from build123d import *

# Parameters (mm, degrees)
F2_W           = 143.0530622602
F2_H           = 41.3108188659
F3_DEPTH       = 14.2
F4_DEPTH       = 45
F5_R           = 3.175
F6_DEPTH       = 25
F7_R           = 11.27
F7_R_2         = 5.0034619329
F8_DEPTH       = 20.6
F9_DEPTH       = 38.1921002041
F11_R          = 5.5610063416
F12_DEPTH      = 13
F13_R          = 3.175
F14_DEPTH      = 25.5131088414
F14_DEPTH_BACK = 25


with BuildPart() as f1:
    # F0 (on Front) → F1 (revolve)
    with BuildSketch(Plane.XZ):
        with BuildLine():
            ThreePointArc((-23.8617697281, 6.3559776459), (-20.6996107179, 0.4699326202), (-16.1176094264, -4.3931980396))
            Line((-16.1176094264, -4.3931980396), (-16.1176094264, 11.4784657965))
            Line((-16.1176094264, 11.4784657965), (0, 11.4784657965))
            Line((0, 11.4784657965), (0, 40.8949155528))
            ThreePointArc((0, 40.8949155528), (-20.9900112333, 29.8840868605), (-23.8617697281, 6.3559776459))
        make_face()
        with BuildLine():
            ThreePointArc((-16.1176094264, -4.3931980396), (-8.5539497274, -8.6525348005), (0, -10.12930213))
            Line((0, -10.12930213), (0, 11.4784657965))
            Line((0, 11.4784657965), (-16.1176094264, 11.4784657965))
            Line((-16.1176094264, 11.4784657965), (-16.1176094264, -4.3931980396))
        make_face()
        with BuildLine():
            Line((-16.1176094264, -14.11514998), (-16.1176094264, -39.7087657565))
            Line((-16.1176094264, -39.7087657565), (0, -39.7087657565))
            Line((0, -39.7087657565), (0, -10.12930213))
            ThreePointArc((0, -10.12930213), (-8.5539497274, -8.6525348005), (-16.1176094264, -4.3931980396))
            Line((-16.1176094264, -4.3931980396), (-16.1176094264, -14.11514998))
        make_face()
        with BuildLine():
            Line((-23.8617697281, 6.3559776459), (-16.1176094264, -14.11514998))
            Line((-16.1176094264, -14.11514998), (-16.1176094264, -4.3931980396))
            ThreePointArc((-16.1176094264, -4.3931980396), (-20.6996107179, 0.4699326202), (-23.8617697281, 6.3559776459))
        make_face()
    revolve(axis=Axis((0, 0, 1.6492682043), (0, 0, -1)))

    # F2 (on Top) → F3 (cut)
    with BuildSketch(Plane.XY):
        with Locations((1.9829161465, 28.7757953629)):
            Rectangle(F2_W, F2_H)
        with Locations((1.9829161465, -28.7757953629)):
            Rectangle(F2_W, F2_H)
    extrude(amount=-F3_DEPTH, mode=Mode.SUBTRACT)

    # F2 (on Top) → F4 (cut)
    with BuildSketch(Plane.XY):
        with Locations((1.9829161465, 28.7757953629)):
            Rectangle(F2_W, F2_H)
        with Locations((1.9829161465, -28.7757953629)):
            Rectangle(F2_W, F2_H)
    extrude(amount=F4_DEPTH, mode=Mode.SUBTRACT)

    # F5 (on face) → F6 (cut)
    with BuildSketch(Plane(origin=(0, 8.1203859299, 0), x_dir=(-1, 0, 0), z_dir=(0, 1, 0))):
        with BuildLine():
            ThreePointArc((4.2365711861, 6.3245803627), (-9.9889031453, 15.8537779996), (5.0700626603, 24.0022303941))
            Line((5.0700626603, 24.0022303941), (9.4230322282, 31.4025509617))
            ThreePointArc((9.4230322282, 31.4025509617), (-18.5650084761, 16.2581366481), (7.8739355899, -1.4524800561))
            Line((7.8739355899, -1.4524800561), (4.2365711861, 6.3245803627))
        make_face()
        with Locations((0, 15.3828067114)):
            Circle(F5_R)
    extrude(amount=-F6_DEPTH, mode=Mode.SUBTRACT)

    # F7 (on face) → F8 (cut)
    with BuildSketch(Plane(origin=(0, 0, -39.7087657565), x_dir=(1, 0, 0), z_dir=(0, 0, -1))):
        Circle(F7_R)
        Circle(F7_R_2, mode=Mode.SUBTRACT)
    extrude(amount=-F8_DEPTH, mode=Mode.SUBTRACT)

    # F7 (on face) → F9 (cut, up to face)
    with BuildSketch(Plane(origin=(0, 0, -39.7087657565), x_dir=(1, 0, 0), z_dir=(0, 0, -1))):
        Circle(F7_R_2)
    extrude(amount=-F9_DEPTH, mode=Mode.SUBTRACT)

    # F11 (on offset) → F12 (cut)
    with BuildSketch(Plane.XY.offset(41.8)):
        Circle(F11_R)
    extrude(amount=-F12_DEPTH, mode=Mode.SUBTRACT)

    # F13 (on Right) → F14 (cut, two sides)
    with BuildSketch(Plane.YZ) as f14_sk:
        with Locations((0, -31.4537657565)):
            Circle(F13_R)
    extrude(amount=F14_DEPTH, mode=Mode.SUBTRACT)
    extrude(f14_sk.sketch, amount=-F14_DEPTH_BACK, mode=Mode.SUBTRACT)


solid = f1.part
Can you work these out from the model? Positions are in its coordinate system, mm. A direction names the side the tool comes from. Coordinates: 2 decimals unless noted, no trailing zeros. Loops run counter-clockwise (first coordinate to the right, second up) from the corner with the lowest first, then second, coordinate; pieces in that order, holes last. Notation, with made-up numbers: (49, -31.75) - (54, -31.75) arc R8 ccw to (54, -19.75) - close; hole circle Ø10 at (88, 36). An arc over 180 degrees is marked (long way). Put each result on its own line as item: value. Start each with the question number.
Item 1: Suppose I cut it at D-D (y = -9.5). Please give me the cut outline in (x, z).
Item 2: If I drill on line 1 along Z through (x, y) = (0, -2); line 2 along Z through (x, y) = (7.5, 5.5); line 3 along Z through (x, y) = (13.1, 0), over which ranges is the centre line in solid material (lowest first)?
Item 3: Suppose I cut it at C-C (z = -5). Please give me the cut outline in (x, y), and give its area (3 significant figures).
Item 4: Suppose I cut it at A-A (y = 0). State how many separate pieces and enclosed holes the cut face has, and give its area (3 significant figures).
Item 5: If we mould it in two halves opening along X, with no side actions, what happens to faces 1 (the face through (-19.935, -0.147, -4.023)), 2 (the face through (10.75, -3.39, -29.55)), 3 (the face through (18.532, 0.114, 16.792)), 4 (the face through (0, -11, -14.2))? For each: +X half, -X half, draft (parallel to the pull), parting line (faces both ways), or undercut.
Item 6: For pin 1 (14.5 mm diameter, centred on x = 0, y = 0, fed in from -Z); pin 2 (7.5 mm diameter, centred on y = 0, z = -31.45, fed in from -X); pin 3 (6.5 mm diameter, centred on x = 3.5, y = 13, fed in from +Z); pin 4 (11.5 mm diameter, centred on x = 0, y = 0, fed in from +Z), each with a flat end and sliding along its axis, tell me the tip position at first contact or that it passes through.
Item 7: Which directions (+Z, -Z, +X, -X, +Y, -Y) give clear straight access to the entire face, cutting with the end or side of a thin tool? Please do faces 5 (the face through (-6, -8.12, 13)), 6 (the face through (-6.08, 0.11, 2.38)), 7 (the face through (-6, 8.12, 13)), 8 (the face through (5, 2, -19.109)).
Here are the results:
1. outline: (-13.02, -39.71) - (-6.06, -39.71) - (-6.06, -19.11) - (6.06, -19.11) - (6.06, -39.71) - (13.02, -39.71) - (13.02, -14.2) - (-13.02, -14.2) - close
2. line 1: 5.38 to 12.21, 18.56 to 25.38
2. line 2: -19.11 to -1.62, 8.77 to 22, 32.39 to 39.14
2. line 3: -39.71 to -34.63, -28.28 to 2.2, 28.57 to 37.27
3. outline: (-17.8, -8.12) - (17.8, -8.12) arc R19.57 ccw to (17.8, 8.12) - (-17.8, 8.12) arc R19.57 ccw to start; hole circle Ø10.01 at (0, 0)
3. area: 538 mm²
4. separate pieces: 4
4. enclosed holes: 1
4. area: 1,820 mm²
5. face 1: -X half
5. face 2: undercut
5. face 3: undercut
5. face 4: draft
6. pin 1: z = -19.11
6. pin 2: x = -16.12
6. pin 3: z = -14.2
6. pin 4: z = 40.28
7. face 5: +Z, +X, -X, -Y
7. face 6: +Y, -Y
7. face 7: +Z, +X, -X, +Y
7. face 8: -Z
